Check sheet for the modelled part. Datum: model origin and axes. Units: mm. Face numbers are marked on the shaded views. A direction names the side the tool comes from. Round coordinates to 2 decimals unless told otherwise and drop trailing zeros. Write each loop counter-clockwise with the first axis right and the second up, starting at its lowest first coordinate (ties: lowest second). Pieces come first, ordered by that corner, then holes. Notation, with made-up numbers: M -5.75,38 L 28.25,38 A28 ccw 28.25,68 Z; hole C 9,13.25 d8. An arc over 180 degrees is marked long. One line per item, written item: value.
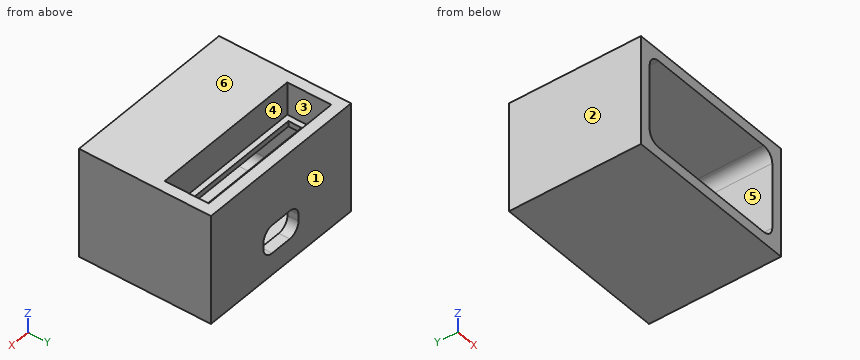
from build123d import *

# Parameters (mm, degrees)
F0_W      = 101.6
F0_H      = 76.2
F1_DEPTH  = 63.5
F3_DEPTH  = 69.85
F4_W      = 88.9
F4_H      = 25.4
F5_DEPTH  = 25.4
F7_DEPTH  = 25.4
F8_W      = 88.9
F8_H      = 3.175
F9_DEPTH  = 31.75
F10_W     = 88.9
F10_H     = 6.35
F11_DEPTH = 19.05
F12_W     = 82.55
F12_H     = 7.62
F13_DEPTH = 25.4


with BuildPart() as f1:
    # F0 (on Top) → F1 (new body)
    with BuildSketch(Plane.XY):
        with Locations((-49.642408, -6.194344)):
            Rectangle(F0_W, F0_H)
    extrude(amount=F1_DEPTH)

    # F2 (on face) → F3 (cut)
    with BuildSketch(Plane.XZ.offset(44.294344)):
        with BuildLine():
            Line((-11.542408, 57.15), (-87.742408, 57.15))
            ThreePointArc((-87.742408, 57.15), (-92.232536, 55.290128), (-94.092408, 50.8))
            Line((-94.092408, 50.8), (-94.092408, 12.7))
            ThreePointArc((-94.092408, 12.7), (-92.232536, 8.209872), (-87.742408, 6.35))
            Line((-87.742408, 6.35), (-11.542408, 6.35))
            ThreePointArc((-11.542408, 6.35), (-7.05228, 8.209872), (-5.192408, 12.7))
            Line((-5.192408, 12.7), (-5.192408, 50.8))
            ThreePointArc((-5.192408, 50.8), (-7.05228, 55.290128), (-11.542408, 57.15))
        make_face()
    extrude(amount=-F3_DEPTH, mode=Mode.SUBTRACT)

    # F4 (on face) → F5 (cut)
    with BuildSketch(Plane.XY.offset(63.5)):
        with Locations((-49.642408, 12.855656)):
            Rectangle(F4_W, F4_H)
    extrude(amount=-F5_DEPTH, mode=Mode.SUBTRACT)

    # F6 (on face) → F7 (cut)
    with BuildSketch(Plane.XZ.offset(-25.555656)):
        with BuildLine():
            Line((-43.292408, 29.21), (-55.992408, 29.21))
            ThreePointArc((-55.992408, 29.21), (-60.482536, 27.350128), (-62.342408, 22.86))
            Line((-62.342408, 22.86), (-62.342408, 19.05))
            ThreePointArc((-62.342408, 19.05), (-60.482536, 14.559872), (-55.992408, 12.7))
            Line((-55.992408, 12.7), (-43.292408, 12.7))
            ThreePointArc((-43.292408, 12.7), (-38.80228, 14.559872), (-36.942408, 19.05))
            Line((-36.942408, 19.05), (-36.942408, 22.86))
            ThreePointArc((-36.942408, 22.86), (-38.80228, 27.350128), (-43.292408, 29.21))
        make_face()
    extrude(amount=-F7_DEPTH, mode=Mode.SUBTRACT)

    # F8 (on face) → F9 (join)
    with BuildSketch(Plane.XZ.offset(-25.555656)):
        with Locations((-49.642408, 42.8625)):
            Rectangle(F8_W, F8_H)
    extrude(amount=F9_DEPTH)

    # F10 (on face) → F11 (join)
    with BuildSketch(Plane.XY.offset(63.5)):
        with Locations((-49.642408, -3.019344)):
            Rectangle(F10_W, F10_H)
    extrude(amount=-F11_DEPTH)

    # F12 (on face) → F13 (cut)
    with BuildSketch(Plane.XY.offset(44.45)):
        with Locations((-49.642408, 7.140656)):
            Rectangle(F12_W, F12_H)
    extrude(amount=-F13_DEPTH, mode=Mode.SUBTRACT)


solid = f1.part
Q1. Scan lines: line 1 (X direction, y = -6, z = 13.5); line 2 (Z direction, x = -26.5, y = -37.5); line 3 (Z direction, x = -14, y = 22) (3 decimals). Record each from-to range of solid material in increasing order. Write a range as [from, to].
Completed:
line 1: [-100.44, -94.09], [-5.19, 1.16]
line 2: [0, 6.35], [57.15, 63.5]
line 3: [0, 6.35], [41.275, 44.45]
Q2. Sectioned sample at B-B on x = -83.5. Enter the section's corners in (y, z) (3 decimals).
Completed:
outline: M -44.294,0 L 31.906,0 L 31.906,63.5 L 25.556,63.5 L 25.556,44.45 L 10.951,44.45 L 10.951,41.275 L 25.556,41.275 L 25.556,6.35 L -44.294,6.35 Z; M -44.294,57.15 L -6.194,57.15 L -6.194,41.275 L 3.331,41.275 L 3.331,44.45 L 0.156,44.45 L 0.156,63.5 L -44.294,63.5 Z
Q3. Access from +Z, -Z, +X, -X, +Y, -Y to the whole of each face (thin tool, end or side, straight path). Record for the marked faces 4, 5 and 6.
Completed:
face 4: +Z
face 5: -Y
face 6: +Z, +X, -X, +Y, -Y
Q4. Sectioned sample at D-D on x = -50. Enter the section's corners in (y, z) (3 decimals), and give its area (3 significant figures).
Completed:
outline: M -44.294,0 L 31.906,0 L 31.906,12.7 L 25.556,12.7 L 25.556,6.35 L -44.294,6.35 Z; M -44.294,57.15 L -6.194,57.15 L -6.194,41.275 L 3.331,41.275 L 3.331,44.45 L 0.156,44.45 L 0.156,63.5 L -44.294,63.5 Z; M 10.951,41.275 L 25.556,41.275 L 25.556,29.21 L 31.906,29.21 L 31.906,63.5 L 25.556,63.5 L 25.556,44.45 L 10.951,44.45 Z
area: 1,180 mm^2
Q5. Sectioned sample at C-C on z = 25.5. Enter the section's corners in (x, y).
Completed:
outline: M -100.44,-44.29 L -94.09,-44.29 L -94.09,25.56 L -61.77,25.56 L -61.77,31.91 L -100.44,31.91 Z; M -37.52,25.56 L -5.19,25.56 L -5.19,-44.29 L 1.16,-44.29 L 1.16,31.91 L -37.52,31.91 Z
Q6. Draft check along X on the marked faces 1, 2 and 3. Enter one of: pulls with the +X half, pulls with the -X half, needs draft (parallel to the pull), parting line crosses it, or undercut.
Completed:
face 1: needs draft
face 2: pulls with the -X half
face 3: undercut
Q7. Depth check by flat-ended pin: P1, Ø12.5, axis at x = -40.5, z = 52, coming from the -Y side; P2, Ø1, axis at x = -62, z = 42.5, coming from the -Y side; P3, Ø20.5, axis at x = -54, y = 10.5, coming from the +Z side; P4, Ø12, axis at x = -22.5, z = 30.5, coming from the -Y side. Enter the tip coordinate at first touch or a pass-through.
Completed:
P1: y = -44.29
P2: y = -6.19
P3: z = 44.45
P4: y = 25.56
Q8. Sectioned sample at A-A on y = 24. Enter the section's corners in (x, z) (3 decimals), and give its area (3 significant figures).
Completed:
outline: M -100.442,0 L 1.158,0 L 1.158,63.5 L -5.192,63.5 L -5.192,44.45 L -94.092,44.45 L -94.092,63.5 L -100.442,63.5 Z; hole M -94.092,12.7 A6.35 ccw -87.742,6.35 L -11.542,6.35 A6.35 ccw -5.192,12.7 L -5.192,41.275 L -94.092,41.275 Z
area: 1,670 mm^2
